```python
from build123d import *

# Parameters (mm, degrees)
SKETCH1_W = 9.525
SKETCH1_H = 9.128125
FILLET1_R = 3.175
FILLET2_R = 0.254


with BuildPart() as part:
    # Sketch1 → Revolve1 (revolve)
    with BuildSketch(Plane(origin=(0, 0, 0), x_dir=(0, 0, -1), z_dir=(1, 0, 0))):
        with Locations((0, 8.1359375)):
            Rectangle(SKETCH1_W, SKETCH1_H)
    revolve(axis=Axis((0, 0, 0), (0, 0, 1)))

    # Fillet1
    fillet1_edges = [part.edges().sort_by_distance(p)[0] for p in [
        (0, -12.7, 4.7625),
        (0, -12.7, -4.7625),
    ]]
    fillet(fillet1_edges, radius=FILLET1_R)

    # Fillet2
    fillet2_edges = [part.edges().sort_by_distance(p)[0] for p in [
        (0, -3.571875, -4.7625),
        (0, -3.571875, 4.7625),
    ]]
    fillet(fillet2_edges, radius=FILLET2_R)


solid = part.part
```
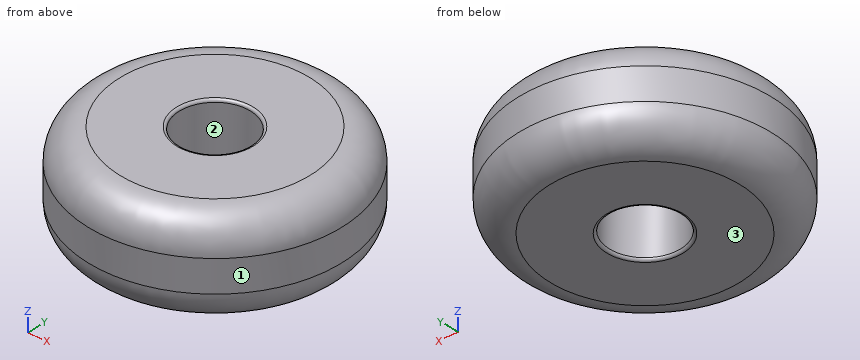
The model under review builds one solid part; all positions refer to its coordinate system, in mm. Face numbers are marked on the shaded views. Round coordinates to 2 decimals unless told otherwise and drop trailing zeros. Loops run counter-clockwise (first coordinate to the right, second up) from the corner with the lowest first, then second, coordinate; pieces in that order, holes last. Notation, with made-up numbers: (20, 82) - (61, 82) arc R11 cw to (61, 89) - close; hole circle Ø5 at (13.25, 76.25). An arc over 180 degrees is marked (long way). Use a Markdown table: item, result. Add a question column.
Q1. Insertion check: pin 1 Ø5 at (y, z) = (-5, -3) entering from -X; pin 2 Ø1.5 at (x, z) = (-1.5, -4) entering from +Y; pin 3 Ø6.5 at (x, y) = (0, 0) entering from -Z; pin 4 Ø5 at (y, z) = (-7, -3.5) entering from -X. Each pin has a flat end and moves straight along its axis. Give the tip position at first contact, or say it passes through.
Q2. Add section D-D (z = -2). State the section outline as (x, y) points.
Q3. Add section C-C (z = -0.25). State the section outline as (x, y) points.
Q4. For probe 1 along Y at (x, z) = (0, 0); probe 2 along Z at (x, y) = (4, 10), list the stretches that pass through material, from the lowest coordinate up.
Q5. The part is to be moulded in two halves that separate along Y. For the marked faces 1, 2 and 3, say which applies: pulls with the +Y half, pulls with the -Y half, needs draft (parallel to the pull), parting line crosses it, or undercut.
Worked answers:
| question | item | result |
|---|---|---|
| 1 | pin 1 | x = -12.38 |
| 1 | pin 2 | y = 12.15 |
| 1 | pin 3 | through |
| 1 | pin 4 | x = -11.67 |
| 2 | outline | circle Ø25.35 at (0, 0); hole circle Ø7.14 at (0, 0) |
| 3 | outline | circle Ø25.4 at (0, 0); hole circle Ø7.14 at (0, 0) |
| 4 | probe 1 | -12.7 to -3.57, 3.57 to 12.7 |
| 4 | probe 2 | -4.51 to 4.51 |
| 5 | face 1 | parting line crosses it |
| 5 | face 2 | undercut |
| 5 | face 3 | needs draft |
